```python
from build123d import *

# Parameters (mm, degrees)
PLATE_SKETCH_W       = 61.5
PLATE_SKETCH_H       = 47
PLATE_DEPTH          = 3.2
POSTS_DEPTH          = 20
SERVO_HOLES_SKETCH_R = 1.6
SERVO_HOLES_DEPTH    = 53.1
PANEL_HOLE_SKETCH_R  = 9.9
PANEL_HOLE_DEPTH     = 18.2


with BuildPart() as part:
    # Plate Sketch → Plate (new body)
    with BuildSketch(Plane(origin=(0, 14, 0), x_dir=(1, 0, 0), z_dir=(0, 1, 0))):
        with Locations((-10, -10.5)):
            Rectangle(PLATE_SKETCH_W, PLATE_SKETCH_H)
    extrude(amount=PLATE_DEPTH)

    # Posts Sketch → Posts (add)
    with BuildSketch(Plane.XY.offset(14)):
        Polygon((-40.75, 17.2), (-38.25, 17.2), (-38.25, 42.6), (-30.5, 42.6), (-30.5, 45.6), (-40.75, 45.6), align=None)
        Polygon((20.75, 17.2), (18.25, 17.2), (18.25, 42.6), (10.5, 42.6), (10.5, 45.6), (20.75, 45.6), align=None)
    extrude(amount=POSTS_DEPTH)

    # Servo Holes Sketch → Servo Holes (cut, symmetric)
    with BuildSketch(Plane(origin=(0, 0, 0), x_dir=(1, 0, 0), z_dir=(0, 1, 0))):
        with Locations(Location((-34.75, -19, 0), (0, 0, 270))):
            Circle(SERVO_HOLES_SKETCH_R)
        with Locations(Location((-34.75, -29, 0), (0, 0, 270))):
            Circle(SERVO_HOLES_SKETCH_R)
        with Locations(Location((14.75, -19, 0), (0, 0, 270))):
            Circle(SERVO_HOLES_SKETCH_R)
        with Locations(Location((14.75, -29, 0), (0, 0, 270))):
            Circle(SERVO_HOLES_SKETCH_R)
    extrude(amount=SERVO_HOLES_DEPTH, both=True, mode=Mode.SUBTRACT)

    # Panel Hole Sketch → Panel Hole (cut, symmetric)
    with BuildSketch(Plane(origin=(0, 0, 0), x_dir=(1, 0, 0), z_dir=(0, 1, 0))):
        with Locations(Location((0, 0, 0), (0, 0, 90))):
            Circle(PANEL_HOLE_SKETCH_R)
    extrude(amount=PANEL_HOLE_DEPTH, both=True, mode=Mode.SUBTRACT)


solid = part.part
```
Could you check a few things on this model? Use its own coordinates, in mm. A direction names the side the tool comes from. Coordinates: 2 decimals unless noted, no trailing zeros. Write each loop counter-clockwise with the first axis right and the second up, starting at its lowest first coordinate (ties: lowest second). Pieces come first, ordered by that corner, then holes. Notation, with made-up numbers: (62, 55) - (73, 55) arc R31 cw to (73, 93) - close; hole circle Ø1 at (-31.5, -13.5). An arc over 180 degrees is marked (long way). Use a Markdown table: item, result.
Q1. I'm going to push flat-ended pins straight in: pin 1 Ø11.5 at (x, y) = (-38, 36) entering from -Z; pin 2 Ø12 at (x, z) = (10.5, -1.5) entering from +Y. Where does each tip first touch, or does it pass through?
Geometry check:
| item | result |
|---|---|
| pin 1 | stops at z = 14 |
| pin 2 | stops at y = 17.2 |
Q2. Imagine slicing it at A-A (y = 21). List the corners of the cut face in (x, z) for me.
Geometry check:
| item | result |
|---|---|
| outline | (-40.75, 14) - (-38.25, 14) - (-38.25, 34) - (-40.75, 34) - close; (18.25, 14) - (20.75, 14) - (20.75, 34) - (18.25, 34) - close |
Q3. Imagine slicing it at B-B (x = 11.5). List the corners of the cut face in (y, z) for me, and give its area (3 significant figures).
Geometry check:
| item | result |
|---|---|
| outline | (14, -13) - (17.2, -13) - (17.2, 34) - (14, 34) - close; (42.6, 14) - (45.6, 14) - (45.6, 34) - (42.6, 34) - close |
| area | 210 mm2 |
Q4. Thinking about a two-plate mould opening in Z: for faces 4 (the flat face through (-40.75, 30, 21)), 5 (the flat face through (-39, 34, 14)), 6 (the cylindrical face through (-36, 16, 28)), which applies, +Z half, -Z half, draft (parallel to the pull), parting line (faces both ways), or undercut?
Geometry check:
| item | result |
|---|---|
| face 4 | draft |
| face 5 | -Z half |
| face 6 | undercut |
Q5. Imagine slicing it at C-C (z = 19). List the corners of the cut face in (x, y) for me, and give its area (3 significant figures).
Geometry check:
| item | result |
|---|---|
| outline | (-40.75, 14) - (-36.35, 14) - (-36.35, 17.2) - (-38.25, 17.2) - (-38.25, 42.6) - (-36.35, 42.6) - (-36.35, 45.6) - (-40.75, 45.6) - close; (-33.15, 14) - (13.15, 14) - (13.15, 17.2) - (-33.15, 17.2) - close; (-33.15, 42.6) - (-30.5, 42.6) - (-30.5, 45.6) - (-33.15, 45.6) - close; (10.5, 42.6) - (13.15, 42.6) - (13.15, 45.6) - (10.5, 45.6) - close; (16.35, 14) - (20.75, 14) - (20.75, 45.6) - (16.35, 45.6) - (16.35, 42.6) - (18.25, 42.6) - (18.25, 17.2) - (16.35, 17.2) - close |
| area | 346 mm2 |
Q6. Please list where these lines run through material, in increasing order: L1, parallel to Z at x = -34.75, y = 43.7; L2, parallel to X at y = 44.75, z = 19; L3, parallel to X at y = 19.5, z = 20.
Geometry check:
| item | result |
|---|---|
| L1 | z = 14 to 17.4, 20.6 to 27.4, 30.6 to 34 |
| L2 | x = -40.75 to -36.35, -33.15 to -30.5, 10.5 to 13.15, 16.35 to 20.75 |
| L3 | x = -40.75 to -38.25, 18.25 to 20.75 |
Q7. Which directions (+Z, -Z, +X, -X, +Y, -Y) give clear straight access to the entire face, cutting with the end or side of a thin tool? Please do faces 1 (the flat face through (18.25, 30, 24)), 2 (the cylindrical face through (16, 44, 18)), 3 (the flat face through (10.5, 44, 24)).
Geometry check:
| item | result |
|---|---|
| face 1 | +Z, -Z |
| face 2 | +Y, -Y |
| face 3 | +Z, -Z, +Y |
Q8. Imagine slicing it at D-D (x = -34.75). List the corners of the cut face in (y, z) for me.
Geometry check:
| item | result |
|---|---|
| outline | (14, -13) - (17.2, -13) - (17.2, 17.4) - (14, 17.4) - close; (14, 20.6) - (17.2, 20.6) - (17.2, 27.4) - (14, 27.4) - close; (14, 30.6) - (17.2, 30.6) - (17.2, 34) - (14, 34) - close; (42.6, 14) - (45.6, 14) - (45.6, 17.4) - (42.6, 17.4) - close; (42.6, 20.6) - (45.6, 20.6) - (45.6, 27.4) - (42.6, 27.4) - close; (42.6, 30.6) - (45.6, 30.6) - (45.6, 34) - (42.6, 34) - close |
